Geometry check sheet. Reference: drawing and pictorial views, mm from the part's lowest x, y, z. Round coordinates to 2 decimals unless told otherwise and drop trailing zeros. Write each loop counter-clockwise with the first axis right and the second up, starting at its lowest first coordinate (ties: lowest second). Pieces come first, ordered by that corner, then holes. Notation, with made-up numbers: (-23.75, 2.25) - (27.25, 2.25) arc R19 ccw to (27.25, 27.25) - close; hole circle Ø5 at (57, 7). An arc over 180 degrees is marked (long way). Return JSON: item names as keys, results as strings.
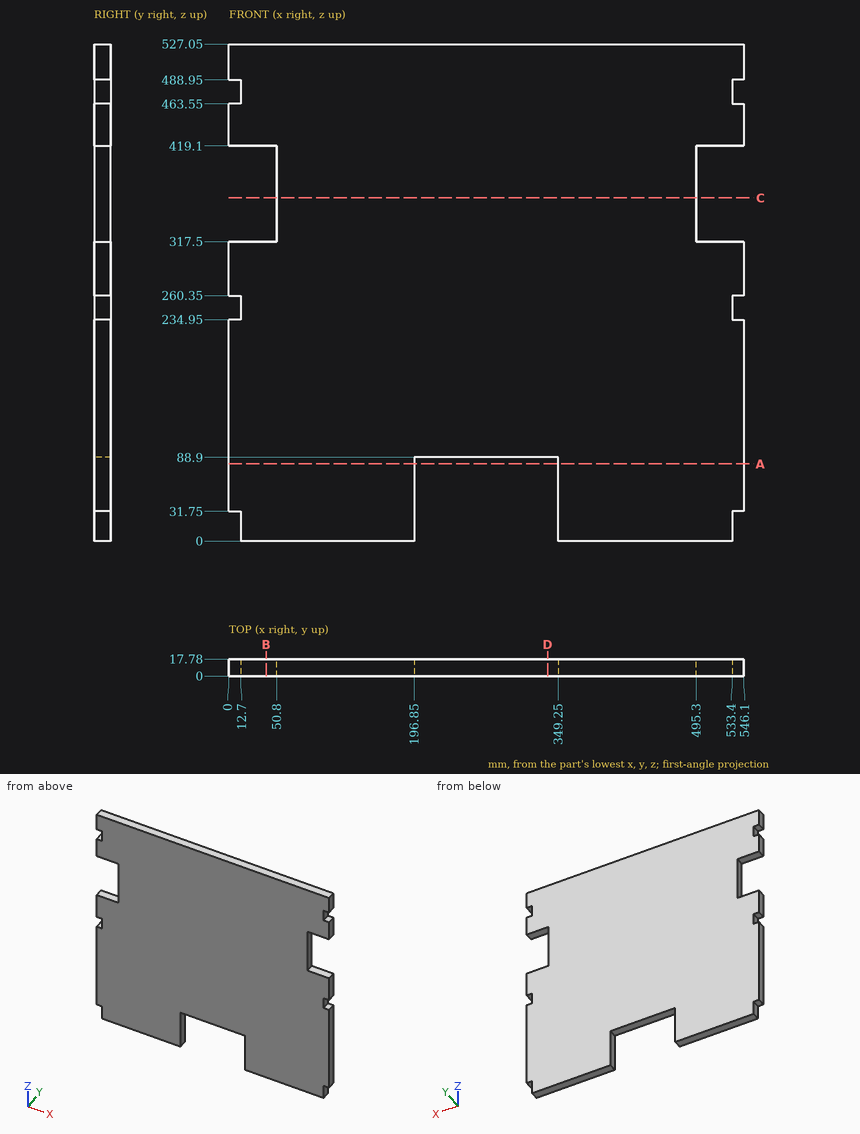
(1) Section check C-C, the plane z = 364. Enter the section's corners in (x, y), plus the area to 3 significant figures.
Response values:
{"outline": "(50.8, 0) - (495.3, 0) - (495.3, 17.78) - (50.8, 17.78) - close", "area": "7,900 mm^2"}
(2) Section check A-A, the plane z = 82. Enter the section's corners in (x, y), plus the area to 3 significant figures.
Response values:
{"outline": "(0, 0) - (196.85, 0) - (196.85, 17.78) - (0, 17.78) - close; (349.25, 0) - (546.1, 0) - (546.1, 17.78) - (349.25, 17.78) - close", "area": "7,000 mm^2"}
(3) Section check D-D, the plane x = 338. Enter the section's corners in (y, z).
Response values:
{"outline": "(0, 88.9) - (17.78, 88.9) - (17.78, 527.05) - (0, 527.05) - close"}
(4) Material ranges on line 1 along X through (y, z) = (10, 66); line 2 along X through (y, z) = (6.25, 332); line 3 along Z through (x, y) = (323, 6.25), recorded low to high. Write a range as [from, to].
Response values:
{"line 1": "x = [0, 196.85], [349.25, 546.1]", "line 2": "x = [50.8, 495.3]", "line 3": "z = [88.9, 527.05]"}
(5) Section check B-B, the plane x = 39.5. Enter the section's corners in (y, z), plus the area to 3 significant figures.
Response values:
{"outline": "(0, 0) - (17.78, 0) - (17.78, 317.5) - (0, 317.5) - close; (0, 419.1) - (17.78, 419.1) - (17.78, 527.05) - (0, 527.05) - close", "area": "7,560 mm^2"}
(6) Gauge pin test, flat ends, axial feed: pin 1 (5.5 mm diameter, centred on y = 10.5, z = 476.5, fed in from +X); pin 2 (5.5 mm diameter, centred on y = 11.5, z = 475, fed in from -X); pin 3 (10 mm diameter, centred on x = 542, y = 10, fed in from -Z). Record the tip position at first contact, or that the pin passes through.
Response values:
{"pin 1": "stops at x = 533.4", "pin 2": "stops at x = 12.7", "pin 3": "stops at z = 31.75"}
